Can you work these out from the model? Positions are in its coordinate system, mm. A direction names the side the tool comes from. Round coordinates to 2 decimals unless told otherwise and drop trailing zeros. Order: outer loops, then holes, each group sorted by start corner. A loop starts at its lowest first (then second) coordinate and runs counter-clockwise, first axis right, second up.
Q1. We'd pull the mould along X, two halves only. Please class faces 1 (the face through (-18, -2, -15.829)), 2 (the face through (1, -2, 15.221)), 3 (the face through (24.974, -2, -2)): pulls with the +X half, pulls with the -X half, needs draft (parallel to the pull), parting line crosses it, or undercut.
Q2. Will these pins go through, and if not, where does the flat tip stop? P1, Ø16, axis at x = -10.5, z = 6.5, coming from the -Y side; P2, Ø1.3, axis at x = 4.5, y = -2.5, coming from the -Z side.
Q3. For faces 4 (the face through (0, -3, -7.079)), 5 (the face through (-4.275, -1.014, 12.05)), 6 (the face through (12.974, -2, -14)), which set-ups out of +Z, -Z, +X, -X, +Y, -Y let a thin tool reach every point of the face, with its end or its side?
Q4. If we section it at C-C (x = 18.5): Please give me the cut outline in (y, z).
Q5. If we section it at B-B (z = -0.5): Please give me the cut outline in (x, y), plus the area to 3 significant figures.
Q6. If we section it at A-A (y = -2.65): Please give me the cut outline in (x, z), plus the area to 3 significant figures.
Q7. If I drill on line 1 (Z direction, x = -16, y = -3.75); line 2 (X direction, y = -4.3, z = -2); line 3 (Z direction, x = -8.5, y = -3), over which ranges is the centre line in solid material (lowest first)?
Q8. If we section it at D-D (x = -10): Please give me the cut outline in (y, z).
from build123d import *

# Parameters (mm, degrees)
F0_W     = 45.2
F0_H     = 20.3
F0_R     = 8.1
F0_W_2   = 10.5
F0_H_2   = 4.8
F1_DEPTH = 2
F0_W_3   = 12
F0_H_3   = 10
F2_DEPTH = 4.5
F3_R     = 2


# Not quite as in the source:
# - a feature names something its author has since deleted; it is built from what else it names


with BuildPart() as f1:
    # F0 (on Front) → F1 (new body)
    with BuildSketch(Plane.XZ):
        with Locations((0.3735902304, 3.0706598967)):
            Rectangle(F0_W, F0_H)
        with Locations((-12.7264097696, 3.0706598967)):
            Circle(F0_R, mode=Mode.SUBTRACT)
        with Locations((0.3735902304, 10.2206598967)):
            Rectangle(F0_W_2, F0_H_2, mode=Mode.SUBTRACT)
        with Locations((13.4735902304, 3.0706598967)):
            Circle(F0_R, mode=Mode.SUBTRACT)
    extrude(amount=F1_DEPTH)



with BuildPart() as f1b:
    # F0 (on Front) → F1, piece 2 (new body)
    with BuildSketch(Plane.XZ):
        with Locations((18.9735902304, -14.0793401033)):
            Rectangle(F0_W_3, F0_H_3)
        with BuildLine():
            ThreePointArc((16.1235902304, -15.8293401033), (14.3735902304, -14.0793401033), (16.1235902304, -12.3293401033))
            Line((16.1235902304, -12.3293401033), (21.8235902304, -12.3293401033))
            ThreePointArc((21.8235902304, -12.3293401033), (23.0610270975, -12.8419032362), (23.5735902304, -14.0793401033))
            ThreePointArc((23.5735902304, -14.0793401033), (23.0610270975, -15.3167769703), (21.8235902304, -15.8293401033))
            Line((21.8235902304, -15.8293401033), (16.1235902304, -15.8293401033))
        make_face(mode=Mode.SUBTRACT)
    extrude(amount=F1_DEPTH)


with BuildPart() as f1_1:
    add(f1.part)

    add(f1b.part)  # F2 merges F1b
    # F0 (on Front) → F2 (join)
    with BuildSketch(Plane.XZ):
        Polygon((24.9735902304, 15.2206598967), (-24.2264097696, 15.2206598967), (-24.2264097696, -9.0793401033), (-12.2264097696, -9.0793401033), (12.9735902304, -9.0793401033), (24.9735902304, -9.0793401033), align=None)
        with Locations((0.3735902304, 3.0706598967)):
            Rectangle(F0_W, F0_H, mode=Mode.SUBTRACT)
        with Locations((-18.2264097696, -14.0793401033)):
            Rectangle(F0_W_3, F0_H_3)
        with BuildLine():
            Line((-21.0764097696, -12.3293401033), (-15.3764097696, -12.3293401033))
            ThreePointArc((-15.3764097696, -12.3293401033), (-14.1389729025, -12.8419032362), (-13.6264097696, -14.0793401033))
            ThreePointArc((-13.6264097696, -14.0793401033), (-14.1389729025, -15.3167769703), (-15.3764097696, -15.8293401033))
            Line((-15.3764097696, -15.8293401033), (-21.0764097696, -15.8293401033))
            ThreePointArc((-21.0764097696, -15.8293401033), (-22.8264097696, -14.0793401033), (-21.0764097696, -12.3293401033))
        make_face(mode=Mode.SUBTRACT)
        with Locations((18.9735902304, -14.0793401033)):
            Rectangle(F0_W_3, F0_H_3)
        with BuildLine():
            ThreePointArc((16.1235902304, -15.8293401033), (14.3735902304, -14.0793401033), (16.1235902304, -12.3293401033))
            Line((16.1235902304, -12.3293401033), (21.8235902304, -12.3293401033))
            ThreePointArc((21.8235902304, -12.3293401033), (23.0610270975, -12.8419032362), (23.5735902304, -14.0793401033))
            ThreePointArc((23.5735902304, -14.0793401033), (23.0610270975, -15.3167769703), (21.8235902304, -15.8293401033))
            Line((21.8235902304, -15.8293401033), (16.1235902304, -15.8293401033))
        make_face(mode=Mode.SUBTRACT)
    extrude(amount=F2_DEPTH)

    # F3
    f3_edges = [f1_1.edges().sort_by_distance(p)[0] for p in [
        (-4.87641, -1, 7.82066),
        (-4.87641, -1, 12.62066),
        (5.62359, -1, 12.62066),
        (5.62359, -1, 7.82066),
    ]]
    fillet(f3_edges, radius=F3_R)


solid = f1_1.part
Solution:
1. face 1: undercut
1. face 2: needs draft
1. face 3: pulls with the +X half
2. P1: stops at y = -4.5
2. P2: stops at z = -9.08
3. face 4: -Y
3. face 5: +Y, -Y
3. face 6: -Z, +Y, -Y
4. outline: (-4.5, -19.08) - (0, -19.08) - (0, -15.83) - (-4.5, -15.83) - close; (-4.5, -12.33) - (0, -12.33) - (0, -3.28) - (-2, -3.28) - (-2, -7.08) - (-4.5, -7.08) - close; (-4.5, 13.22) - (-2, 13.22) - (-2, 9.42) - (0, 9.42) - (0, 15.22) - (-4.5, 15.22) - close
5. outline: (-24.23, -4.5) - (-22.23, -4.5) - (-22.23, -2) - (-20, -2) - (-20, 0) - (-24.23, 0) - close; (-5.46, -2) - (6.2, -2) - (6.2, 0) - (-5.46, 0) - close; (20.74, -2) - (22.97, -2) - (22.97, -4.5) - (24.97, -4.5) - (24.97, 0) - (20.74, 0) - close
5. area: 50.2 mm2
6. outline: (-24.23, -19.08) - (-12.23, -19.08) - (-12.23, -9.08) - (12.97, -9.08) - (12.97, -19.08) - (24.97, -19.08) - (24.97, 15.22) - (-24.23, 15.22) - close; hole (-22.23, -7.08) - (22.97, -7.08) - (22.97, 13.22) - (-22.23, 13.22) - close; hole (-21.08, -15.83) - (-15.38, -15.83) arc R1.75 ccw to (-15.38, -12.33) - (-21.08, -12.33) arc R1.75 ccw to start; hole (16.12, -15.83) - (21.82, -15.83) arc R1.75 ccw to (21.82, -12.33) - (16.12, -12.33) arc R1.75 ccw to start
6. area: 459 mm2
7. line 1: z = -19.08 to -15.83, -12.33 to -7.08, 13.22 to 15.22
7. line 2: x = -24.23 to -22.23, 22.97 to 24.97
7. line 3: z = -9.08 to -7.08, 13.22 to 15.22
8. outline: (-4.5, -9.08) - (0, -9.08) - (0, -4.56) - (-2, -4.56) - (-2, -7.08) - (-4.5, -7.08) - close; (-4.5, 13.22) - (-2, 13.22) - (-2, 10.7) - (0, 10.7) - (0, 15.22) - (-4.5, 15.22) - close
